```python
from build123d import *

# Parameters (mm, degrees)
F0_R          = 12.5
F1_DEPTH      = 3
F2_R          = 12
F3_DEPTH      = 1.666667
F4_R          = 12.5
F4_R_2        = 12
F5_DEPTH      = 2.5
F5_DEPTH_BACK = 0.5


with BuildPart() as f1:
    # F0 (on Front) → F1 (new body)
    with BuildSketch(Plane.XZ):
        with Locations((-48.996713, 23.240132)):
            Circle(F0_R)
    extrude(amount=F1_DEPTH)

    # F2 (on face) → F3 (join)
    with BuildSketch(Plane.XZ.offset(3)):
        with Locations((-48.997421, 23.245247)):
            Circle(F2_R)
    extrude(amount=F3_DEPTH)

    # F4 (on face) → F5 (join, two sides)
    with BuildSketch(Plane.XZ.offset(4.666667)) as f5_sk:
        with Locations((-48.997421, 23.245247)):
            Circle(F4_R)
        with Locations((-48.997421, 23.245247)):
            Circle(F4_R_2, mode=Mode.SUBTRACT)
        with Locations((-48.997421, 23.245247)):
            Circle(F4_R_2)
    extrude(amount=F5_DEPTH)
    extrude(f5_sk.sketch, amount=-F5_DEPTH_BACK)


solid = f1.part
```
Here's how the part is built. I have some questions about the finished solid (model axes, mm). Coordinates: 2 decimals unless noted, no trailing zeros. Write each loop counter-clockwise with the first axis right and the second up, starting at its lowest first coordinate (ties: lowest second). Pieces come first, ordered by that corner, then holes. Notation, with made-up numbers: (26, 8) -> (77, 8) arc R13 ccw to (77, 33) -> close; hole circle Ø5 at (43.25, 21). An arc over 180 degrees is marked (long way). Use a Markdown table: item, result. Add a question column.
(1) If we section it at C-C, the plane y = -6.25: Write out the boundary of the cut face in (x, z), and give its area (3 significant figures).
(2) Please list where these lines run through material, in increasing order: line 1 (Z direction, x = -46.5, y = -3.25); line 2 (Z direction, x = -41.5, y = -4.5); line 3 (X direction, y = -1.75, z = 19).
(3) I'm going to push flat-ended pins straight in: P1, Ø2, axis at x = -46.5, y = -3, coming from the +Z side; P2, Ø1, axis at y = -2, z = 19.5, coming from the +X side. Where does each tip first touch, or does it pass through?
(4) If we section it at B-B, the plane x = -38.25: Write out the boundary of the cut face in (y, z).
(5) We'd pull the mould along Y, two halves only. Please class faces 1 (the flat face through (-49, -7.167, 23)), 2 (the cylindrical face through (-58.2, -1.5, 31.7)), 3 (the cylindrical face through (-37.91, -3.58, 18.65)), 4 (the flat face through (-55.54, -4.167, 33.49)): +Y half, -Y half, draft (parallel to the pull), parting line (faces both ways), or undercut.
(6) If we section it at A-A, the plane z = 16.25: Write out the boundary of the cut face in (x, y), and give its area (3 significant figures).
Outcome:
| question | item | result |
|---|---|---|
| 1 | outline | circle Ø25 at (-49, 23.25) |
| 1 | area | 491 mm^2 |
| 2 | line 1 | z = 11.51 to 34.98 |
| 2 | line 2 | z = 13.24 to 33.25 |
| 2 | line 3 | x = -60.76 to -37.24 |
| 3 | P1 | stops at z = 35.65 |
| 3 | P2 | stops at x = -36.92 |
| 4 | outline | (-7.17, 16.86) -> (-4.17, 16.86) -> (-4.17, 17.91) -> (-3, 17.91) -> (-3, 16.86) -> (0, 16.86) -> (0, 29.62) -> (-3, 29.62) -> (-3, 28.58) -> (-4.17, 28.58) -> (-4.17, 29.63) -> (-7.17, 29.63) -> close |
| 5 | face 1 | -Y half |
| 5 | face 2 | draft |
| 5 | face 3 | undercut |
| 5 | face 4 | undercut |
| 6 | outline | (-59.36, -7.17) -> (-38.64, -7.17) -> (-38.64, -4.17) -> (-39.25, -4.17) -> (-39.25, -3) -> (-38.63, -3) -> (-38.63, 0) -> (-59.36, 0) -> (-59.36, -3) -> (-58.75, -3) -> (-58.75, -4.17) -> (-59.36, -4.17) -> close |
| 6 | area | 147 mm^2 |
